```python
from build123d import *

# Parameters (mm, degrees)
SKETCH1_R           = 12.5
BOSS_EXTRUDE1_DEPTH = 10


with BuildPart() as part:
    # Sketch1 → Boss-Extrude1 (new body)
    with BuildSketch(Plane.XY):
        with BuildLine():
            Line((-25, 0), (-45, 0))
            ThreePointArc((-45, 0), (-52.071067812, -2.928932188), (-55, -10))
            Line((-55, -10), (-55, -30))
            Line((-55, -30), (95, -30))
            Line((95, -30), (65, 0))
            Line((65, 0), (25, 0))
            ThreePointArc((25, 0), (0, 25), (-25, 0))
        make_face()
        Circle(SKETCH1_R, mode=Mode.SUBTRACT)
    extrude(amount=BOSS_EXTRUDE1_DEPTH)


solid = part.part
```
Geometry check sheet. Reference: the model listing, model coordinates, mm. A direction names the side the tool comes from. Give positions to 0.01 mm unless a question says otherwise; leave off trailing zeros. Write each loop counter-clockwise with the first axis right and the second up, starting at its lowest first coordinate (ties: lowest second). Pieces come first, ordered by that corner, then holes.
1) Release check for a two-part mould opening along X. For faces 1 (the flat face through (80, -15, 5)), 2 (the cylindrical face through (11.923, 3.755, 4.93)), 3 (the flat face through (45, 0, 5)) record: pulls with the +X half, pulls with the -X half, needs draft (parallel to the pull), parting line crosses it, or undercut.
2) Section check B-B, the plane z = 5.5. Record the boundary of the cut face in (x, y), and give its area (3 significant figures).
3) Material ranges on L1, parallel to Y at x = 0, z = 5; L2, parallel to Y at x = 59, z = 8.25; L3, parallel to X at y = -4, z = 8, recorded low to high.
4) Section check C-C, the plane y = 20. Record the boundary of the cut face in (x, z), and give its area (3 significant figures).
5) Section check A-A, the plane x = 0. Record the boundary of the cut face in (y, z), and give its area (3 significant figures).
6) Section check D-D, the plane x = 70. Record the boundary of the cut face in (y, z).
7) Access from +Z, -Z, +X, -X, +Y, -Y to the whole of each face (thin tool, end or side, straight path). Record for faces 4 (the flat face through (-35, 0, 5)), 5 (the flat face through (2, -14, 10)).
8) Gauge pin test, flat ends, axial feed: pin 1 (1 mm diameter, centred on y = -5, z = 5.5, fed in from +X); pin 2 (6 mm diameter, centred on y = 11.5, z = 2, fed in from -X); pin 3 (5 mm diameter, centred on x = -24.5, z = 1.5, fed in from +Y). Record the tip position at first contact, or that the pin passes through.
Computed:
1. face 1: pulls with the +X half
1. face 2: undercut
1. face 3: needs draft
2. outline: (-55, -30) - (95, -30) - (65, 0) - (25, 0) arc R25 ccw to (-25, 0) - (-45, 0) arc R10 ccw to (-55, -10) - close; hole circle Ø25 at (0, 0)
2. area: 4,520 mm2
3. L1: y = -30 to -12.5, 12.5 to 25
3. L2: y = -30 to 0
3. L3: x = -53 to -11.84, 11.84 to 69
4. outline: (-15, 0) - (15, 0) - (15, 10) - (-15, 10) - close
4. area: 300 mm2
5. outline: (-30, 0) - (-12.5, 0) - (-12.5, 10) - (-30, 10) - close; (12.5, 0) - (25, 0) - (25, 10) - (12.5, 10) - close
5. area: 300 mm2
6. outline: (-30, 0) - (-5, 0) - (-5, 10) - (-30, 10) - close
7. face 4: +Z, -Z, -X, +Y
7. face 5: +Z, +X, -X, +Y, -Y
8. pin 1: stops at x = 70.5
8. pin 2: stops at x = -23.51
8. pin 3: stops at y = 11.87
